Geometry check sheet. Reference: the model listing, model coordinates, mm. Face numbers are marked on the shaded views. A direction names the side the tool comes from. Round coordinates to 2 decimals unless told otherwise and drop trailing zeros. Order: outer loops, then holes, each group sorted by start corner. A loop starts at its lowest first (then second) coordinate and runs counter-clockwise, first axis right, second up.
```python
from build123d import *

# Parameters (mm, degrees)
F0_W     = 220.749088
F0_H     = 102.985457
F1_DEPTH = 39.5
F2_W     = 198.709123
F2_H     = 81.303883
F3_DEPTH = 38.2
F5_D     = 5.5


with BuildPart() as f1:
    # F0 (on Top) → F1 (new body)
    with BuildSketch(Plane.XY):
        with Locations((10.852728, -7.735457)):
            Rectangle(F0_W, F0_H)
    extrude(amount=F1_DEPTH)

    # F2 (on face) → F3 (cut)
    with BuildSketch(Plane.XY.offset(39.5)):
        with Locations((10.40272, -7.478898)):
            Rectangle(F2_W, F2_H)
    extrude(amount=-F3_DEPTH, mode=Mode.SUBTRACT)

    # F5 (through all)
    with Locations(Plane.XZ.offset(59.228186)):
        with Locations((-83.465457, 6.931819), (104.943641, 6.704546)):
            Hole(F5_D / 2)


solid = f1.part
```
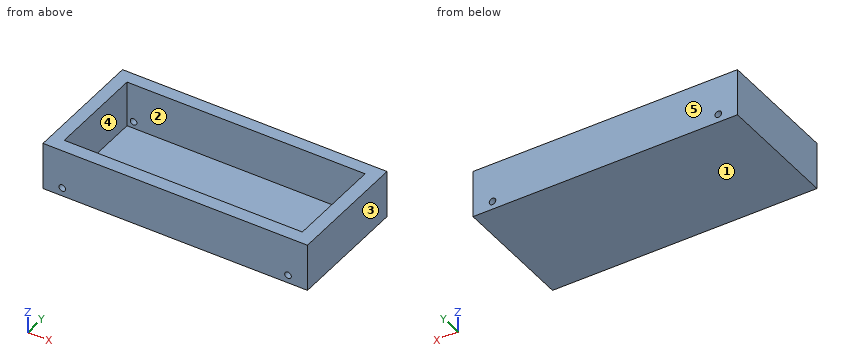
(1) Draft check along X on the marked faces 1, 2 and 3. Enter one of: released by +X, released by -X, zero draft, split by the parting line, or undercut.
Returned:
face 1: zero draft
face 2: undercut
face 3: released by +X
(2) Depth check by flat-ended pin: P1, Ø1.5, axis at x = 94, y = -3.5, coming from the +Z side. Enter the tip coordinate at first touch or a pass-through.
Returned:
P1: stops at z = 1.3
(3) Sectioned sample at C-C, the plane x = 45.5. Record the cut outline in (y, z).
Returned:
outline: (-59.23, 0) - (43.76, 0) - (43.76, 39.5) - (33.17, 39.5) - (33.17, 1.3) - (-48.13, 1.3) - (-48.13, 39.5) - (-59.23, 39.5) - close
(4) Sectioned sample at A-A, the plane z = 26. Record the cut outline in (x, y), and give its area (3 significant figures).
Returned:
outline: (-99.52, -59.23) - (121.23, -59.23) - (121.23, 43.76) - (-99.52, 43.76) - close; hole (-88.95, -48.13) - (109.76, -48.13) - (109.76, 33.17) - (-88.95, 33.17) - close
area: 6,580 mm2
(5) Material ranges on line 1 (X direction, y = -16, z = 12); line 2 (Y direction, x = -2, z = 32.5); line 3 (Z direction, x = -70, y = -44), recorded low to high.
Returned:
line 1: x = -99.52 to -88.95, 109.76 to 121.23
line 2: y = -59.23 to -48.13, 33.17 to 43.76
line 3: z = 0 to 1.3
(6) Sectioned sample at B-B, the plane y = 11. Record the cut outline in (x, z).
Returned:
outline: (-99.52, 0) - (121.23, 0) - (121.23, 39.5) - (109.76, 39.5) - (109.76, 1.3) - (-88.95, 1.3) - (-88.95, 39.5) - (-99.52, 39.5) - close
(7) Set-up check for the marked faces 4 and 5: record each of +Z, -Z, +X, -X, +Y, -Y from which the full face is reachable in a straight line by a thin tool's end or side.
Returned:
face 4: +Z
face 5: +Z, -Z, +X, -X, +Y
